```python
from build123d import *

# Parameters (mm, degrees)
ESQUISSE1_W             = 38
ESQUISSE1_H             = 320
BOSS_EXTRU_1_DEPTH      = 3
ENL_V_MAT_EXTRU_1_REACH = 192.418
ESQUISSE2_R             = 2
ENL_V_MAT_EXTRU_2_REACH = 192.418
ESQUISSE3_W             = 38
ESQUISSE3_H             = 236


with BuildPart() as part:
    # Esquisse1 → Boss.-Extru.1 (new body)
    with BuildSketch(Plane.XY):
        with Locations((76, 5)):
            Rectangle(ESQUISSE1_W, ESQUISSE1_H)
    extrude(amount=BOSS_EXTRU_1_DEPTH)

    # Esquisse2 → Enlèv. mat.-Extru.1 (cut, up to next)
    with BuildSketch(Plane.XY.offset(3), mode=Mode.PRIVATE) as enl_v_mat_extru_1_sk1:
        with Locations((73, 155)):
            Circle(ESQUISSE2_R)
    enl_v_mat_extru_1_tool1 = extrude(enl_v_mat_extru_1_sk1.sketch, amount=-ENL_V_MAT_EXTRU_1_REACH, mode=Mode.PRIVATE) & part.part
    # Esquisse2 → Enlèv. mat.-Extru.1 (cut, up to next)
    with BuildSketch(Plane.XY.offset(3), mode=Mode.PRIVATE) as enl_v_mat_extru_1_sk2:
        with Locations((79, 97)):
            Circle(ESQUISSE2_R)
    enl_v_mat_extru_1_tool2 = extrude(enl_v_mat_extru_1_sk2.sketch, amount=-ENL_V_MAT_EXTRU_1_REACH, mode=Mode.PRIVATE) & part.part
    add(enl_v_mat_extru_1_tool1.solids().sort_by_distance((73, 155, 3))[0], mode=Mode.SUBTRACT)
    add(enl_v_mat_extru_1_tool2.solids().sort_by_distance((79, 97, 3))[0], mode=Mode.SUBTRACT)

    # Esquisse3 → Enlèv. mat.-Extru.2 (cut, up to next)
    with BuildSketch(Plane.XY.offset(3), mode=Mode.PRIVATE) as enl_v_mat_extru_2_sk1:
        with Locations((76, -37)):
            Rectangle(ESQUISSE3_W, ESQUISSE3_H)
    enl_v_mat_extru_2_tool1 = extrude(enl_v_mat_extru_2_sk1.sketch, amount=-ENL_V_MAT_EXTRU_2_REACH, mode=Mode.PRIVATE) & part.part
    add(enl_v_mat_extru_2_tool1.solids().sort_by_distance((76, -37, 3))[0], mode=Mode.SUBTRACT)


solid = part.part
```
Model file for the job. Use its own axes, mm. Coordinates: 2 decimals unless noted, no trailing zeros. Loops run counter-clockwise (first coordinate to the right, second up) from the corner with the lowest first, then second, coordinate; pieces in that order, holes last. Notation, with made-up numbers: (75, -29.5) - (126, -29.5) arc R12 ccw to (126, -25.5) - close; hole circle Ø8 at (-20.75, 33). An arc over 180 degrees is marked (long way). Answer as a JSON object with one key per item and string values. Group by question number.
(1) Probe line 1 along X through (y, z) = (155, 0.6); line 2 along Y through (x, z) = (79, 2.2); line 3 along Y through (x, z) = (73, 0.75). List the from-to ranges inside material, lowest first.
(2) Cut at A-A (x = 73). Give the cut face in (y, z), then the cut area to 3 significant figures.
(3) Cut at B-B (y = 155). Give the cut face in (x, z).
(4) Two-plate mould, pull along X, no slides. Class faces 1 (the face through (76, 81, 2)), 2 (the face through (95, 122, 1)), 3 (the face through (80.075, 98.686, 1.521)), 4 (the face through (73.923, 153.226, 1.521)): released by +X, released by -X, zero draft, split by the parting line, or undercut.
Geometry says:
{
 "1": {"line 1": "x = 57 to 71, 75 to 95", "line 2": "y = 81 to 95, 99 to 165", "line 3": "y = 81 to 153, 157 to 165"},
 "2": {"outline": "(81, 0) - (153, 0) - (153, 3) - (81, 3) - close; (157, 0) - (165, 0) - (165, 3) - (157, 3) - close", "area": "240 mm^2"},
 "3": {"outline": "(57, 0) - (71, 0) - (71, 3) - (57, 3) - close; (75, 0) - (95, 0) - (95, 3) - (75, 3) - close"},
 "4": {"face 1": "zero draft", "face 2": "released by +X", "face 3": "undercut", "face 4": "undercut"}
}
